Geometry: final body of the model. Coordinates: model frame, mm. Face numbers are marked on the shaded views. A direction names the side the tool comes from. Round coordinates to 2 decimals unless told otherwise and drop trailing zeros. Loops run counter-clockwise (first coordinate to the right, second up) from the corner with the lowest first, then second, coordinate; pieces in that order, holes last. Notation, with made-up numbers: (35.5, 72) - (54.5, 72) arc R21 cw to (54.5, 108) - close; hole circle Ø11 at (7, -10). An arc over 180 degrees is marked (long way). Answer as CSV lines item,"result".
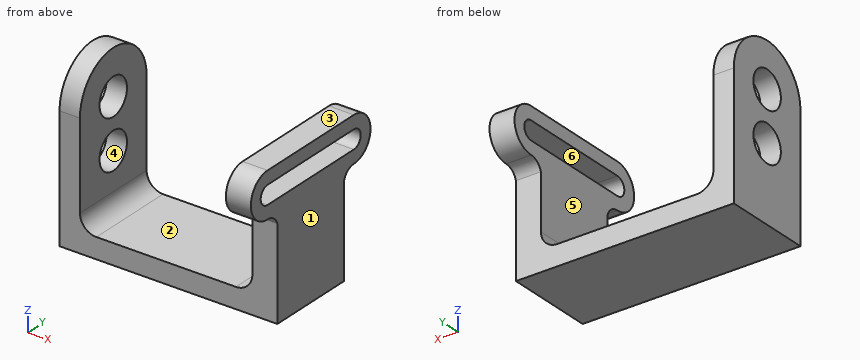
from build123d import *

# Parameters (mm, degrees)
F1_DEPTH = 34.544
F2_W     = 34.544
F2_H     = 3.556
F3_DEPTH = 9.652
F4_DEPTH = 9.652
F6_DEPTH = 7.874
F5_R     = 7.112
F7_DEPTH = 7.874


with BuildPart() as f1:
    # F0 (on Front) → F1 (new body)
    with BuildSketch(Plane.XZ):
        with BuildLine():
            Line((0, 47.752), (0, 0))
            Line((0, 0), (84.074, 0))
            Line((84.074, 0), (84.074, 47.752))
            Line((84.074, 47.752), (74.422, 47.752))
            Line((74.422, 47.752), (74.422, 14.224))
            ThreePointArc((74.422, 14.224), (72.562128, 9.733872), (68.072, 7.874))
            Line((68.072, 7.874), (14.224, 7.874))
            ThreePointArc((14.224, 7.874), (9.733872, 9.733872), (7.874, 14.224))
            Line((7.874, 14.224), (7.874, 47.752))
            Line((7.874, 47.752), (0, 47.752))
        make_face()
    extrude(amount=F1_DEPTH)

    # F2 (on face) → F3 (cut)
    with BuildSketch(Plane.YZ.offset(84.074)):
        with Locations((-17.272, 45.974)):
            Rectangle(F2_W, F2_H)
        with BuildLine():
            Line((-34.544, 44.196), (-39.624, 44.196))
            ThreePointArc((-39.624, 44.196), (-43.18, 47.752), (-39.624, 51.308))
            Line((-39.624, 51.308), (5.08, 51.308))
            ThreePointArc((5.08, 51.308), (8.636, 47.752), (5.08, 44.196))
            Line((5.08, 44.196), (0, 44.196))
            Line((0, 44.196), (0, 39.116))
            Line((0, 39.116), (5.08, 39.116))
            ThreePointArc((5.08, 39.116), (13.716, 47.752), (5.08, 56.388))
            Line((5.08, 56.388), (-39.624, 56.388))
            ThreePointArc((-39.624, 56.388), (-48.26, 47.752), (-39.624, 39.116))
            Line((-39.624, 39.116), (-34.544, 39.116))
            Line((-34.544, 39.116), (-34.544, 44.196))
        make_face()
    extrude(amount=-F3_DEPTH, mode=Mode.SUBTRACT)

    # F2 (on face) → F4 (join)
    with BuildSketch(Plane.YZ.offset(84.074)):
        with BuildLine():
            Line((-34.544, 44.196), (-39.624, 44.196))
            ThreePointArc((-39.624, 44.196), (-43.18, 47.752), (-39.624, 51.308))
            Line((-39.624, 51.308), (5.08, 51.308))
            ThreePointArc((5.08, 51.308), (8.636, 47.752), (5.08, 44.196))
            Line((5.08, 44.196), (0, 44.196))
            Line((0, 44.196), (0, 39.116))
            Line((0, 39.116), (5.08, 39.116))
            ThreePointArc((5.08, 39.116), (13.716, 47.752), (5.08, 56.388))
            Line((5.08, 56.388), (-39.624, 56.388))
            ThreePointArc((-39.624, 56.388), (-48.26, 47.752), (-39.624, 39.116))
            Line((-39.624, 39.116), (-34.544, 39.116))
            Line((-34.544, 39.116), (-34.544, 44.196))
        make_face()
        with BuildLine():
            Line((-34.544, 35.408394), (-34.544, 39.116))
            Line((-34.544, 39.116), (-39.624, 39.116))
            ThreePointArc((-39.624, 39.116), (-36.479451, 38.090523), (-34.544, 35.408394))
        make_face()
        with BuildLine():
            Line((5.08, 39.116), (0, 39.116))
            Line((0, 39.116), (0, 35.408394))
            ThreePointArc((0, 35.408394), (1.935451, 38.090523), (5.08, 39.116))
        make_face()
    extrude(amount=-F4_DEPTH)

    # F5 (on face) → F6 (join)
    with BuildSketch(Plane(origin=(0, 0, 0), x_dir=(0, -1, 0), z_dir=(-1, 0, 0))):
        with BuildLine():
            Line((24.384, 47.752), (34.544, 47.752))
            ThreePointArc((34.544, 47.752), (17.272, 65.024), (0, 47.752))
            Line((0, 47.752), (10.16, 47.752))
            ThreePointArc((10.16, 47.752), (17.272, 54.864), (24.384, 47.752))
        make_face()
    extrude(amount=-F6_DEPTH)

    # F5 (on face) → F7 (cut)
    with BuildSketch(Plane(origin=(0, 0, 0), x_dir=(0, -1, 0), z_dir=(-1, 0, 0))):
        with Locations((17.272, 47.752)):
            Circle(F5_R)
        with Locations((17.272, 28.702)):
            Circle(F5_R)
    extrude(amount=-F7_DEPTH, mode=Mode.SUBTRACT)


solid = f1.part
(1) Access query for the marked faces 4, 5 and 6. Directions: +Z, -Z, +X, -X, +Y, -Y. A direction counts if a zero-diameter tool reaches every point of the face in a straight line with its end or side. Return the directions, or none.
Findings below:
face 4,"-X"
face 5,"+Z, +Y, -Y"
face 6,"+X"
(2) Pin query (flat end, axial travel): P1, Ø10, axis at y = -6, z = 45.5, coming from the -X side; P2, Ø5, axis at x = 78, y = -12.5, coming from the +Z side; P3, Ø10.5, axis at x = 31, y = -16, coming from the +Z side. Return the tip coordinate at first contact, or that it passes through.
Findings below:
P1,"x = 0"
P2,"z = 56.39"
P3,"z = 7.87"
(3) Draft query along X for the marked faces 1, 2 and 3. Return one class per face: pulls with the +X half, pulls with the -X half, needs draft (parallel to the pull), parting line crosses it, or undercut.
Findings below:
face 1,"pulls with the +X half"
face 2,"undercut"
face 3,"needs draft"
(4) Section A-A (y = -16.5). Output: boundary loops of the cut face in (x, z).
Findings below:
outline,"(0, 0) - (84.07, 0) - (84.07, 44.2) - (74.42, 44.2) - (74.42, 14.22) arc R6.35 cw to (68.07, 7.87) - (14.22, 7.87) arc R6.35 cw to (7.87, 14.22) - (7.87, 21.63) - (0, 21.63) - close; (0, 35.77) - (7.87, 35.77) - (7.87, 40.68) - (0, 40.68) - close; (0, 54.82) - (7.87, 54.82) - (7.87, 65.01) - (0, 65.01) - close; (74.42, 51.31) - (84.07, 51.31) - (84.07, 56.39) - (74.42, 56.39) - close"
(5) Material intervals for line 1 along X through (y, z) = (-3.5, 24.5); line 2 along X through (y, z) = (-14, 10); line 3 along Z through (x, y) = (42, -8.5), sorted ascending.
Findings below:
line 1,"0 to 7.87, 74.42 to 84.07"
line 2,"0 to 9.48, 72.81 to 84.07"
line 3,"0 to 7.87"
(6) Section C-C (x = 51). Output: boundary loops of the cut face in (y, z), and give its area (3 significant figures).
Findings below:
outline,"(-34.54, 0) - (0, 0) - (0, 7.87) - (-34.54, 7.87) - close"
area,"272 mm2"
(7) Section B-B (y = -32.5). Output: boundary loops of the cut face in (x, z), and give its area (3 significant figures).
Findings below:
outline,"(0, 0) - (84.07, 0) - (84.07, 44.2) - (74.42, 44.2) - (74.42, 14.22) arc R6.35 cw to (68.07, 7.87) - (14.22, 7.87) arc R6.35 cw to (7.87, 14.22) - (7.87, 55.9) - (0, 55.9) - close; (74.42, 51.31) - (84.07, 51.31) - (84.07, 56.39) - (74.42, 56.39) - close"
area,"1,460 mm2"
(8) Section D-D (x = 6.5). Output: boundary loops of the cut face in (y, z).
Findings below:
outline,"(-34.54, 0) - (0, 0) - (0, 47.75) arc R17.27 ccw to (-34.54, 47.75) - close; hole circle Ø14.22 at (-17.27, 28.7); hole circle Ø14.22 at (-17.27, 47.75)"
